Can you work these out from the drawing? Everything is in mm from the part's minimum corner. A direction names the side the tool comes from. Coordinates: 2 decimals unless noted, no trailing zeros. Loops run counter-clockwise (first coordinate to the right, second up) from the corner with the lowest first, then second, coordinate; pieces in that order, holes last.
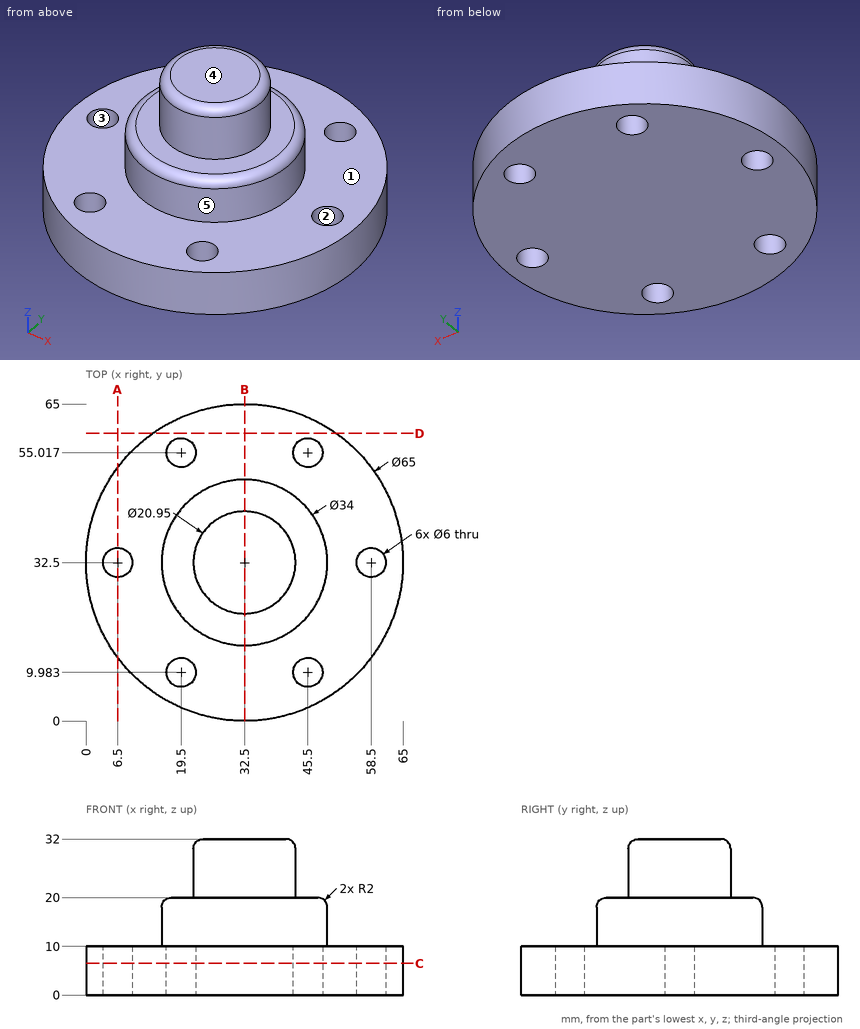
(1) For pin 1 (6 mm diameter, centred on x = 57, y = 39, fed in from +Z); pin 2 (19.5 mm diameter, centred on x = 30.5, y = 23, fed in from +Z); pin 3 (1.5 mm diameter, centred on y = 40, z = 15, fed in from +X); pin 4 (8 mm diameter, centred on x = 22, z = 9.5, fed in from -Y), each with a flat end and sliding along its axis, tell me the tip position at first contact or that it passes through.
Answers:
pin 1: stops at z = 10
pin 2: stops at z = 32
pin 3: stops at x = 48.1
pin 4: stops at y = 0.66
(2) I need wall thicknesses on probe 1 along Y at (x, z) = (45.5, 2); probe 2 along Y at (x, z) = (43, 5) (1 decimal); probe 3 along X at (y, z) = (32, 7). Which ranges of each line are inside material? Lowest first, please.
Answers:
probe 1: y = 2.71 to 6.98, 12.98 to 52.02, 58.02 to 62.29
probe 2: y = 1.7 to 8.3, 11.6 to 53.4, 56.7 to 63.3
probe 3: x = 0 to 3.54, 9.46 to 55.54, 61.46 to 65
(3) Imagine slicing it at B-B, the plane x = 32.5. Write out the boundary of the cut face in (y, z) (1 decimal), and give its area (3 significant figures).
Answers:
outline: (0, 0) - (65, 0) - (65, 10) - (49.5, 10) - (49.5, 18) arc R2 ccw to (47.5, 20) - (43, 20) - (43, 30) arc R2 ccw to (41, 32) - (24, 32) arc R2 ccw to (22, 30) - (22, 20) - (17.5, 20) arc R2 ccw to (15.5, 18) - (15.5, 10) - (0, 10) - close
area: 1,240 mm2
(4) Imagine slicing it at A-A, the plane x = 6.5. Write out the boundary of the cut face in (y, z).
Answers:
outline: (13, 0) - (29.5, 0) - (29.5, 10) - (13, 10) - close; (35.5, 0) - (52, 0) - (52, 10) - (35.5, 10) - close
(5) Imagine slicing it at D-D, the plane y = 59. Write out the boundary of the cut face in (x, z) (1 decimal).
Answers:
outline: (13.7, 0) - (51.3, 0) - (51.3, 10) - (13.7, 10) - close
(6) We'd pull the mould along X, two halves only. Please class the marked faces 3, 4 and 5: +X half, -X half, draft (parallel to the pull), parting line (faces both ways), or undercut.
Answers:
face 3: undercut
face 4: draft
face 5: parting line
(7) Imagine slicing it at C-C, the plane z = 6.5. Write out the boundary of the cut face in (x, y), and give its area (3 significant figures).
Answers:
outline: circle Ø65 at (32.5, 32.5); hole circle Ø6 at (6.5, 32.5); hole circle Ø6 at (19.5, 9.98); hole circle Ø6 at (19.5, 55.02); hole circle Ø6 at (45.5, 9.98); hole circle Ø6 at (45.5, 55.02); hole circle Ø6 at (58.5, 32.5)
area: 3,150 mm2
(8) Which directions (+Z, -Z, +X, -X, +Y, -Y) give clear straight access to the entire face, cutting with the end or side of a thin tool? Please do the marked faces 1 and 2.
Answers:
face 1: +Z
face 2: +Z, -Z
